from build123d import *

# Parameters (mm, degrees)
SKETCH1_R           = 1.75
SKETCH1_R_2         = 1.5
BOSS_EXTRUDE1_DEPTH = 6
MOVE_FACE1_BY       = 0.08
MOVE_FACE1_2_BY     = 0.08
MOVE_FACE1_3_BY     = 0.08
MOVE_FACE1_4_BY     = 0.08
MOVE_FACE1_5_BY     = 0.08


with BuildPart() as part:
    # Sketch1 → Boss-Extrude1 (new body)
    with BuildSketch(Plane.XY):
        with BuildLine():
            ThreePointArc((-24.743686063, 12), (0, -27.5), (24.743686063, 12))
            ThreePointArc((24.743686063, 12), (19.411906952, 15.339946038), (14.08012784, 12))
            ThreePointArc((14.08012784, 12), (0, -18.5), (-14.08012784, 12))
            ThreePointArc((-14.08012784, 12), (-19.411906952, 15.339946038), (-24.743686063, 12))
        make_face()
        with Locations((0, -23)):
            Circle(SKETCH1_R, mode=Mode.SUBTRACT)
        with Locations((-16.263455967, -16.263455967)):
            Circle(SKETCH1_R_2, mode=Mode.SUBTRACT)
        with Locations((-23, 0)):
            Circle(SKETCH1_R, mode=Mode.SUBTRACT)
        with Locations((23, 0)):
            Circle(SKETCH1_R, mode=Mode.SUBTRACT)
        with Locations((16.263455967, -16.263455967)):
            Circle(SKETCH1_R_2, mode=Mode.SUBTRACT)
    extrude(amount=BOSS_EXTRUDE1_DEPTH)

    # Move Face1: a curved face moved outward by 0.08
    add(Solid.thicken(part.faces().sort_by_distance((-24.75, 0, 3))[0], MOVE_FACE1_BY))

    # Move Face1 2: a curved face moved outward by 0.08
    add(Solid.thicken(part.faces().sort_by_distance((-1.75, -23, 3))[0], MOVE_FACE1_2_BY))

    # Move Face1 3: a curved face moved outward by 0.08
    add(Solid.thicken(part.faces().sort_by_distance((-17.763455967, -16.263455967, 3))[0], MOVE_FACE1_3_BY))

    # Move Face1 4: a curved face moved outward by 0.08
    add(Solid.thicken(part.faces().sort_by_distance((21.25, 0, 3))[0], MOVE_FACE1_4_BY))

    # Move Face1 5: a curved face moved outward by 0.08
    add(Solid.thicken(part.faces().sort_by_distance((14.763455967, -16.263455967, 3))[0], MOVE_FACE1_5_BY))


solid = part.part
Verification items for the finished model (mm, model axes). Give positions to 0.01 mm unless a question says otherwise; leave off trailing zeros. Loops run counter-clockwise (first coordinate to the right, second up) from the corner with the lowest first, then second, coordinate; pieces in that order, holes last.
1. Material ranges on probe 1 along Y at (x, z) = (0, 2.6); probe 2 along X at (y, z) = (-16, 5.5); probe 3 along Y at (x, z) = (-16.5, 2.75), recorded low to high.
Derived:
probe 1: y = -27.5 to -24.67, -21.33 to -18.5
probe 2: x = -22.37 to -17.66, -14.87 to -9.29, 9.29 to 14.87, 17.66 to 22.37
probe 3: y = -22 to -17.66, -14.86 to -8.37, 8.37 to 14.58
2. Go/stop test with flat-tipped pins: P1, Ø1, axis at y = -21.5, z = 1.5, coming from the +X side; P2, Ø3, axis at y = -10, z = 1, coming from the -X side. Record where each tip stops, or that it passes through.
Derived:
P1: stops at x = 17.76
P2: stops at x = -26.15
3. Release check for a two-part mould opening along X. For faces 1 (the cylindrical face through (-19.32, 15.34, 2.96)), 2 (the cylindrical face through (-0.78, -27.49, 2.96)), 3 (the flat face through (0, -20, 0)) record: +X half, -X half, draft (parallel to the pull), parting line (faces both ways), or undercut.
Derived:
face 1: undercut
face 2: parting line
face 3: draft
4. Cross-section at C-C on y = -8. Record the cut outline in (x, z), and give its area (3 significant figures).
Derived:
outline: (-26.31, 0) - (-16.68, 0) - (-16.68, 6) - (-26.31, 6) - close; (16.68, 0) - (26.31, 0) - (26.31, 6) - (16.68, 6) - close
area: 116 mm2
5. Cross-section at A-A on x = 0. Record the cut outline in (y, z), and give its area (3 significant figures).
Derived:
outline: (-27.5, 0) - (-24.67, 0) - (-24.67, 6) - (-27.5, 6) - close; (-21.33, 0) - (-18.5, 0) - (-18.5, 6) - (-21.33, 6) - close
area: 34.0 mm2
6. Cross-section at B-B on y = 0. Record the cut outline in (x, z).
Derived:
outline: (-27.5, 0) - (-24.67, 0) - (-24.67, 6) - (-27.5, 6) - close; (-21.33, 0) - (-18.5, 0) - (-18.5, 6) - (-21.33, 6) - close; (18.5, 0) - (21.33, 0) - (21.33, 6) - (18.5, 6) - close; (24.67, 0) - (27.5, 0) - (27.5, 6) - (24.67, 6) - close
7. Cross-section at D-D on z = 3.75. Record the cut outline in (x, y), and give its area (3 significant figures).
Derived:
outline: (-24.74, 12) arc R27.5 ccw (long way) to (24.74, 12) arc R5.93 ccw to (14.08, 12) arc R18.5 cw (long way) to (-14.08, 12) arc R5.93 ccw to start; hole circle Ø3.34 at (-23, 0); hole circle Ø2.84 at (-16.26, -16.26); hole circle Ø3.34 at (0, -23); hole circle Ø2.84 at (16.26, -16.26); hole circle Ø3.34 at (23, 0)
area: 890 mm2
